Work out the finished part from the listing and answer in its coordinate system (mm). Round coordinates to 2 decimals unless told otherwise and drop trailing zeros. Order: outer loops, then holes, each group sorted by start corner. A loop starts at its lowest first (then second) coordinate and runs counter-clockwise, first axis right, second up. Notation, with made-up numbers: (-23, 86.25) - (36, 86.25) arc R19 ccw to (36, 113.25) - close; hole circle Ø8 at (84.25, 26.5). An arc over 180 degrees is marked (long way). Use one line per item in the form item = value. Start each with the question number.
Q1. Given P1, Ø1.5, axis at x = 8.5, z = 1.5, coming from the +Y side, flat-ended and moving along its own axis, determine where the tip first touches the part or whether it passes through.
Q2. Find the intervals of material crossed by line 1 (Y direction, x = 0, z = 1.2); line 2 (X direction, y = -9.5, z = 0.9); line 3 (Y direction, x = -7.75, z = 2.15), in increasing order. Write a range as [from, to].
Q3. The part is cut by section B-B on y = -10. Determine the outline of the cut face in (x, z).
Q4. The part is cut by section D-D on x = -9. Determine the outline of the cut face in (y, z), plus the area to 3 significant figures.
Q5. The part is cut by section A-A on x = 0. Determine the outline of the cut face in (y, z), plus the area to 4 significant figures.
Q6. For a pull along Y with two mould halves and no side action, classify faces 1 (the cylindrical face through (0, 30, 1)), 2 (the cylindrical face through (-10.2, -10.9, 1.5)), 3 (the flat face through (-12.5, 0, 1)), 4 (the cylindrical face through (10.2, -9.1, 1.5)) as +Y half, -Y half, draft (parallel to the pull), parting line (faces both ways), or undercut.
Q7. The part is cut by section C-C on z = 1.3. Determine the outline of the cut face in (x, y), plus the area to 3 significant figures.
from build123d import *

# Parameters (mm, degrees)
EXTRUDE_1_DEPTH     = 3
SKETCH_3_R          = 4
CUT_EXTRUDE_1_DEPTH = 33.638167841
SKETCH_4_R          = 1.5
CUT_EXTRUDE_2_DEPTH = 33.638167841


with BuildPart() as part:
    # 草图2 → 凸台-拉伸1 (new body)
    with BuildSketch(Plane.XY):
        with BuildLine():
            Line((-12.5, 17.5), (-12.5, -17.5))
            Line((-12.5, -17.5), (12.5, -17.5))
            Line((12.5, -17.5), (12.5, 17.5))
            ThreePointArc((12.5, 17.5), (0, 30), (-12.5, 17.5))
        make_face()
    extrude(amount=EXTRUDE_1_DEPTH)

    # 草图3 → 切除-拉伸1 (cut, through all)
    with BuildSketch(Plane.XY.offset(3)):
        with Locations((0, 17.5)):
            Circle(SKETCH_3_R)
    extrude(amount=-CUT_EXTRUDE_1_DEPTH, mode=Mode.SUBTRACT)

    # 草图4 → 切除-拉伸2 (cut, through all)
    with BuildSketch(Plane.XY.offset(3)):
        with Locations((-9, -10)):
            Circle(SKETCH_4_R)
        with Locations((0, -10)):
            Circle(SKETCH_4_R)
        with Locations(Location((9, -10, 0), (0, 0, 180))):
            Circle(SKETCH_4_R)
    extrude(amount=-CUT_EXTRUDE_2_DEPTH, mode=Mode.SUBTRACT)


solid = part.part
Found:
q1.P1 = 27.31
q2.line_1 = [-17.5, -11.5], [-8.5, 13.5], [21.5, 30]
q2.line_2 = [-12.5, -10.41], [-7.59, -1.41], [1.41, 7.59], [10.41, 12.5]
q2.line_3 = [-17.5, -10.83], [-9.17, 27.31]
q3.outline = (-12.5, 0) - (-10.5, 0) - (-10.5, 3) - (-12.5, 3) - close; (-7.5, 0) - (-1.5, 0) - (-1.5, 3) - (-7.5, 3) - close; (1.5, 0) - (7.5, 0) - (7.5, 3) - (1.5, 3) - close; (10.5, 0) - (12.5, 0) - (12.5, 3) - (10.5, 3) - close
q4.outline = (-17.5, 0) - (-11.5, 0) - (-11.5, 3) - (-17.5, 3) - close; (-8.5, 0) - (26.17, 0) - (26.17, 3) - (-8.5, 3) - close
q4.area = 122 mm²
q5.outline = (-17.5, 0) - (-11.5, 0) - (-11.5, 3) - (-17.5, 3) - close; (-8.5, 0) - (13.5, 0) - (13.5, 3) - (-8.5, 3) - close; (21.5, 0) - (30, 0) - (30, 3) - (21.5, 3) - close
q5.area = 109.5 mm²
q6.face_1 = +Y half
q6.face_2 = undercut
q6.face_3 = draft
q6.face_4 = undercut
q7.outline = (-12.5, -17.5) - (12.5, -17.5) - (12.5, 17.5) arc R12.5 ccw to (-12.5, 17.5) - close; hole circle Ø3 at (-9, -10); hole circle Ø8 at (0, 17.5); hole circle Ø3 at (0, -10); hole circle Ø3 at (9, -10)
q7.area = 1,050 mm²
